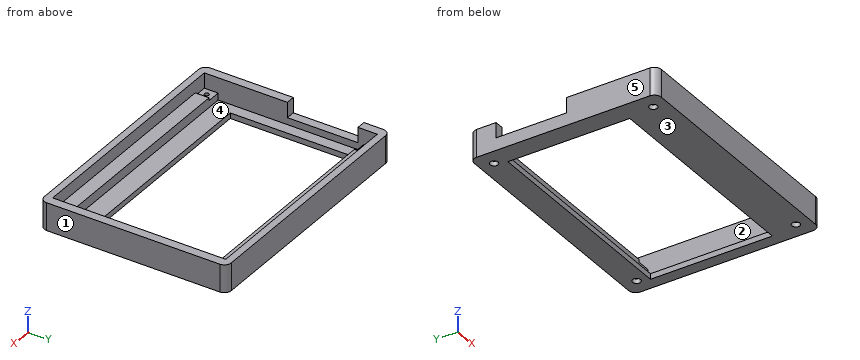
Solid Edge part; units mm, degrees
sketch "Sketch1" plane through (0, 0, 0) normal (0, 0, 1) x (1, 0, 0)
  line L0 (92.7483, 63.0331) -> (-87.2517, 63.0331)
  line L1 (-87.2517, 63.0331) -> (-87.2517, -71.9669)
  line L2 (-87.2517, -71.9669) -> (92.7483, -71.9669)
  line L3 (92.7483, -71.9669) -> (92.7483, 63.0331)
extrude "Protrusion1" add sketch "Sketch1" along normal blind 20
sketch "Sketch2" plane through (2.7483, -4.4669, 20) normal (0, 0, 1) x (1, 0, 0)
  line L0 (-83.5, 62.5) -> (-83.5, -62.5)
  line L1 (83.5, -62.5) -> (-83.5, -62.5)
  line L2 (83.5, -62.5) -> (83.5, 62.5)
  line L3 (83.5, 62.5) -> (-83.5, 62.5)
extrude "ExtrudedCutout_2" cut sketch "Sketch2" against normal blind 9
sketch "Sketch3" plane through (2.7483, -4.4669, 11) normal (0, 0, 1) x (1, 0, 0)
  line L0 (73.5, 52.5) -> (-73.5, 52.5)
  line L1 (-73.5, 52.5) -> (-73.5, 62.5)
  line L2 (-73.5, 62.5) -> (-83.5, 62.5)
  line L3 (-83.5, 62.5) -> (-83.5, -62.5)
  line L4 (-83.5, -62.5) -> (-73.5, -62.5)
  line L5 (-73.5, -62.5) -> (-73.5, -52.5)
  line L6 (-73.5, -52.5) -> (73.5, -52.5)
  line L7 (73.5, -62.5) -> (73.5, -52.5)
  line L8 (83.5, -62.5) -> (73.5, -62.5)
  line L9 (83.5, 62.5) -> (83.5, -62.5)
  line L10 (73.5, 62.5) -> (83.5, 62.5)
  line L11 (73.5, 62.5) -> (73.5, 52.5)
extrude "ExtrudedCutout_3" cut sketch "Sketch3" against normal blind 2
sketch "Sketch4" plane through (2.7483, -4.4669, 11) normal (0, 0, 1) x (1, 0, 0)
  circle A0 centre (-78.5, 57.5) radius 1.6
  circle A1 centre (-78.5, -57.5) radius 1.6
  circle A2 centre (78.5, 57.5) radius 1.6
  circle A3 centre (78.5, -57.5) radius 1.6
extrude "Cutout1" cut sketch "Sketch4" against normal up to next
sketch "Sketch5" plane through (2.7483, -4.4669, 9) normal (0, 0, 1) x (1, 0, 0)
  line L0 (-83.5, 52.5) -> (83.5, 52.5)
  line L1 (83.5, 52.5) -> (83.5, -52.5)
  line L2 (83.5, -52.5) -> (-83.5, -52.5)
  line L3 (-83.5, -52.5) -> (-83.5, 52.5)
extrude "ExtrudedCutout_6" cut sketch "Sketch5" against normal blind 5
sketch "Sketch6" plane through (2.7483, -4.4669, 9) normal (0, 0, 1) x (1, 0, 0)
  line L0 (-75.5, 49.5) -> (81.5, 49.5)
  line L1 (81.5, 49.5) -> (81.5, -38.5)
  line L2 (81.5, -38.5) -> (-75.5, -38.5)
  line L3 (-75.5, -38.5) -> (-75.5, 49.5)
extrude "Cutout2" cut sketch "Sketch6" against normal through all
sketch "Sketch7" plane through (-80.7517, -4.4669, 12) normal (1, 0, 0) x (0, -1, 0)
  line L0 (-48.5, 3) -> (2.5, 3)
  line L1 (2.5, 3) -> (2.5, -8)
  line L2 (2.5, -8) -> (-48.5, -8)
  line L3 (-48.5, 3) -> (-48.5, -8)
extrude "Cutout3" cut sketch "Sketch7" against normal through all
sketch "Sketch8" plane through (2.7483, -4.4669, 0) normal (0, 0, -1) x (-1, 0, 0)
  circle A0 centre (-78.5, 57.5) radius 2.845
  circle A1 centre (-78.5, -57.5) radius 2.845
  circle A2 centre (78.5, -57.5) radius 2.845
  circle A3 centre (78.5, 57.5) radius 2.845
extrude "ExtrudedCutout_10" cut sketch "Sketch8" against normal blind 3.3
fillet "Round_1" radius 5 4 edges at (-87.2517, -71.9669, 10) (92.7483, -71.9669, 10) (92.7483, 63.0331, 10) (-87.2517, 63.0331, 10)
Verification items for the finished model (mm, model axes). Face numbers are marked on the shaded views. A direction names the side the tool comes from. Give positions to 0.01 mm unless a question says otherwise; leave off trailing zeros. Write each loop counter-clockwise with the first axis right and the second up, starting at its lowest first coordinate (ties: lowest second). Pieces come first, ordered by that corner, then holes. Notation, with made-up numbers: (-5, 36) - (29, 36) arc R14 cw to (29, 57) - close; hole circle Ø2 at (64, 10). An arc over 180 degrees is marked (long way). Put each result on its own line as item: value.
Q1. Section check D-D on z = 17.75. Record the cut outline in (x, y).
Result:
outline: (-87.25, -66.97) arc R5 ccw to (-82.25, -71.97) - (87.75, -71.97) arc R5 ccw to (92.75, -66.97) - (92.75, 58.03) arc R5 ccw to (87.75, 63.03) - (-82.25, 63.03) arc R5 ccw to (-87.25, 58.03) - (-87.25, 44.03) - (-80.75, 44.03) - (-80.75, 58.03) - (86.25, 58.03) - (86.25, -66.97) - (-80.75, -66.97) - (-80.75, -6.97) - (-87.25, -6.97) - close
Q2. Scan lines: probe 1 along X at (y, z) = (-57.5, 10); probe 2 along X at (y, z) = (-48.5, 13.25); probe 3 along X at (y, z) = (42.5, 1.5). Record each from-to range of solid material in increasing order. Write a range as from..to.
Result:
probe 1: -87.25..-80.75, -70.75..76.25, 86.25..92.75
probe 2: -87.25..-80.75, 86.25..92.75
probe 3: -87.25..-72.75, 84.25..92.75
Q3. Section check C-C on z = 6.5. Record the cut outline in (x, y).
Result:
outline: (-87.25, -66.97) arc R5 ccw to (-82.25, -71.97) - (87.75, -71.97) arc R5 ccw to (92.75, -66.97) - (92.75, 58.03) arc R5 ccw to (87.75, 63.03) - (-82.25, 63.03) arc R5 ccw to (-87.25, 58.03) - close; hole (-80.75, -56.97) - (86.25, -56.97) - (86.25, 48.03) - (-80.75, 48.03) - close; hole circle Ø3.2 at (-75.75, -61.97); hole circle Ø3.2 at (-75.75, 53.03); hole circle Ø3.2 at (81.25, -61.97); hole circle Ø3.2 at (81.25, 53.03)
Q4. Set-up check for the marked faces 1 and 2: record each of +Z, -Z, +X, -X, +Y, -Y from which the full face is reachable in a straight line by a thin tool's end or side.
Result:
face 1: +Z, -Z, +X, +Y, -Y
face 2: +Z
Q5. Section check A-A on y = -35. Record the cut outline in (x, z).
Result:
outline: (-87.25, 0) - (-72.75, 0) - (-72.75, 4) - (-80.75, 4) - (-80.75, 20) - (-87.25, 20) - close; (84.25, 0) - (92.75, 0) - (92.75, 20) - (86.25, 20) - (86.25, 4) - (84.25, 4) - close
Q6. Mould release check, pull along X, two halves, no side actions. Record for the marked faces 3, 4 and 5: released by +X, released by -X, zero draft, split by the parting line, or undercut.
Result:
face 3: zero draft
face 4: undercut
face 5: released by -X
Q7. Depth check by flat-ended pin: P1, Ø1.5, axis at y = 32, z = 11, coming from the -X side; P2, Ø7, axis at x = -84, y = 10.5, coming from the +Z side; P3, Ø2.5, axis at x = -75.75, y = -61.97, coming from the +Z side. Enter the tip coordinate at first touch or a pass-through.
Result:
P1: x = 86.25
P2: z = 9
P3: through
Q8. Section check B-B on x = -48.5. Record the cut outline in (y, z), and give its area (3 significant figures).
Result:
outline: (-71.97, 0) - (-42.97, 0) - (-42.97, 4) - (-56.97, 4) - (-56.97, 11) - (-66.97, 11) - (-66.97, 20) - (-71.97, 20) - close; (45.03, 0) - (63.03, 0) - (63.03, 20) - (58.03, 20) - (58.03, 11) - (48.03, 11) - (48.03, 4) - (45.03, 4) - close
area: 488 mm2
